```python
from build123d import *

# Parameters (mm, degrees)
SKETCH_1_R          = 25
SKETCH_1_R_2        = 2.55
EXTRUDE_1_DEPTH     = 2
SKETCH_3_R          = 2.05
SKETCH_3_W          = 8.8
SKETCH_3_H          = 2.8
SKETCH_3_W_2        = 2.8
SKETCH_3_H_2        = 8.8
CUT_EXTRUDE_2_DEPTH = 4
SKETCH_7_R          = 3
CUT_EXTRUDE_3_DEPTH = 10
EXTRUDE_3_DEPTH     = 2


with BuildPart() as part:
    # 草图1 → 凸台-拉伸1 (new body)
    with BuildSketch(Plane.XY):
        Polygon((151.457142857, -41.187142857), (151.457142857, 108.812857143), (-148.542857143, 108.812857143), (-148.542857143, -191.187142857), (151.457142857, -191.187142857), align=None)
        with Locations((1.457142857, -41.187142857)):
            Circle(SKETCH_1_R, mode=Mode.SUBTRACT)
        with Locations((25.027142857, -17.617142857)):
            Circle(SKETCH_1_R_2, mode=Mode.SUBTRACT)
        with Locations((25.027142857, -64.757142857)):
            Circle(SKETCH_1_R_2, mode=Mode.SUBTRACT)
        with Locations((-22.112857143, -64.757142857)):
            Circle(SKETCH_1_R_2, mode=Mode.SUBTRACT)
        with Locations((-22.112857143, -17.617142857)):
            Circle(SKETCH_1_R_2, mode=Mode.SUBTRACT)
    extrude(amount=EXTRUDE_1_DEPTH)

    # 草图3 → 切除-拉伸2 (cut)
    with BuildSketch(Plane.XY.offset(2)):
        with Locations((1.457142857, -185.187142857)):
            Circle(SKETCH_3_R)
        with Locations((67.457142857, -185.187142857)):
            Circle(SKETCH_3_R)
        with Locations((-64.542857143, -185.187142857)):
            Circle(SKETCH_3_R)
        with Locations((-142.542857143, 24.812857143)):
            Circle(SKETCH_3_R)
        with Locations((-142.542857143, -41.187142857)):
            Circle(SKETCH_3_R)
        with Locations((-142.542857143, -107.187142857)):
            Circle(SKETCH_3_R)
        with Locations((67.457142857, 102.812857143)):
            Circle(SKETCH_3_R)
        with Locations((1.457142857, 102.812857143)):
            Circle(SKETCH_3_R)
        with Locations((-64.542857143, 102.812857143)):
            Circle(SKETCH_3_R)
        with Locations((145.457142857, -107.187142857)):
            Circle(SKETCH_3_R)
        with Locations((145.457142857, -41.187142857)):
            Circle(SKETCH_3_R)
        with Locations((145.457142857, 24.812857143)):
            Circle(SKETCH_3_R)
        with Locations((50.957142857, -170.187142857)):
            Circle(SKETCH_3_R)
        with Locations((-48.042857143, -170.187142857)):
            Circle(SKETCH_3_R)
        with Locations((1.457142857, -88.187142857)):
            Circle(SKETCH_3_R)
        with Locations((-31.776875859, -74.421161573)):
            Circle(SKETCH_3_R)
        with Locations((-45.542857143, -41.187142857)):
            Circle(SKETCH_3_R)
        with Locations((-31.776875859, -7.953124141)):
            Circle(SKETCH_3_R)
        with Locations((1.457142857, 5.812857143)):
            Circle(SKETCH_3_R)
        with Locations((34.691161573, -7.953124141)):
            Circle(SKETCH_3_R)
        with Locations((48.457142857, -41.187142857)):
            Circle(SKETCH_3_R)
        with Locations((34.691161573, -74.421161573)):
            Circle(SKETCH_3_R)
        with Locations((1.457142857, -125.187142857)):
            Circle(SKETCH_3_R)
        with Locations((100.457142857, -185.187142857)):
            Rectangle(SKETCH_3_W, SKETCH_3_H)
        with Locations((34.457142857, -185.187142857)):
            Rectangle(SKETCH_3_W, SKETCH_3_H)
        with Locations((-31.542857143, -185.187142857)):
            Rectangle(SKETCH_3_W, SKETCH_3_H)
        with Locations((-97.542857143, -185.187142857)):
            Rectangle(SKETCH_3_W, SKETCH_3_H)
        with Locations((-142.542857143, 57.812857143)):
            Rectangle(SKETCH_3_W_2, SKETCH_3_H_2)
        with Locations((-142.542857143, -8.187142857)):
            Rectangle(SKETCH_3_W_2, SKETCH_3_H_2)
        with Locations((-142.542857143, -74.187142857)):
            Rectangle(SKETCH_3_W_2, SKETCH_3_H_2)
        with Locations((-142.542857143, -140.187142857)):
            Rectangle(SKETCH_3_W_2, SKETCH_3_H_2)
        with Locations((100.457142857, 102.812857143)):
            Rectangle(SKETCH_3_W, SKETCH_3_H)
        with Locations((34.457142857, 102.812857143)):
            Rectangle(SKETCH_3_W, SKETCH_3_H)
        with Locations((-31.542857143, 102.812857143)):
            Rectangle(SKETCH_3_W, SKETCH_3_H)
        with Locations((-97.542857143, 102.812857143)):
            Rectangle(SKETCH_3_W, SKETCH_3_H)
        with Locations((145.457142857, -140.187142857)):
            Rectangle(SKETCH_3_W_2, SKETCH_3_H_2)
        with Locations((145.457142857, -74.187142857)):
            Rectangle(SKETCH_3_W_2, SKETCH_3_H_2)
        with Locations((145.457142857, -8.187142857)):
            Rectangle(SKETCH_3_W_2, SKETCH_3_H_2)
        with Locations((145.457142857, 57.812857143)):
            Rectangle(SKETCH_3_W_2, SKETCH_3_H_2)
    extrude(amount=-CUT_EXTRUDE_2_DEPTH, mode=Mode.SUBTRACT)

    # 草图7 → 切除-拉伸3 (cut)
    with BuildSketch(Plane.XY.offset(2)):
        with Locations((-88.542857143, -171.187142857)):
            Circle(SKETCH_7_R)
        with Locations((91.457142857, -171.187142857)):
            Circle(SKETCH_7_R)
        with Locations((-128.542857143, 48.812857143)):
            Circle(SKETCH_7_R)
        with Locations((-128.542857143, -131.187142857)):
            Circle(SKETCH_7_R)
        with Locations((91.457142857, 88.812857143)):
            Circle(SKETCH_7_R)
        with Locations((-88.542857143, 88.812857143)):
            Circle(SKETCH_7_R)
        with Locations((131.457142857, -131.187142857)):
            Circle(SKETCH_7_R)
        with Locations((131.457142857, 48.812857143)):
            Circle(SKETCH_7_R)
    extrude(amount=-CUT_EXTRUDE_3_DEPTH, mode=Mode.SUBTRACT)

    # 草图9 → 凸台-拉伸3 (add)
    with BuildSketch(Plane.XY.offset(2)):
        Polygon((151.457142857, 108.812857143), (251.457142857, 108.812857143), (251.457142857, -191.187142857), (251.457142857, -231.187142857), (-148.542857143, -231.187142857), (-148.542857143, -191.187142857), (151.457142857, -191.187142857), align=None)
    extrude(amount=-EXTRUDE_3_DEPTH)


solid = part.part
```
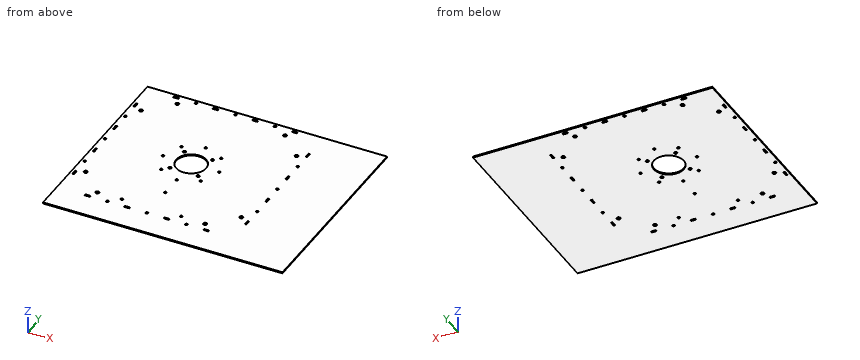
Here's how the part is built. I have some questions about the finished solid (model axes, mm). Coordinates: 2 decimals unless noted, no trailing zeros. Answer as a JSON object with one key per item and string values. Group by question number.
(1) For pin 1 (5.5 mm diameter, centred on x = -142.54, y = -107.19, fed in from -Z); pin 2 (3.5 mm diameter, centred on x = 145.46, y = -107.19, fed in from +Z), each with a flat end and sliding along its axis, tell me the tip position at first contact or that it passes through.
(2) Suppose I cut it at A-A, the plane z = 0.4. State how many separate pieces and enclosed holes the cut face has, then the cut area to 3 significant figures.
(3) I need wall thicknesses on probe 1 along Y at (x, z) = (97, 0.2); probe 2 along X at (y, z) = (58.5, 1.15); probe 3 along X at (y, z) = (6, 0.7). Which ranges of each line are inside material? Lowest first, please.
Values found:
{
 "1": {"pin 1": "stops at z = 0", "pin 2": "passes through"},
 "2": {"separate pieces": "1", "enclosed holes": "52", "area": "133,000 mm^2"},
 "3": {"probe 1": "y = -231.19 to -186.59, -183.79 to 101.41, 104.21 to 108.81", "probe 2": "x = -148.54 to -143.94, -141.14 to 144.06, 146.86 to 251.46", "probe 3": "x = -148.54 to -0.58, 3.5 to 251.46"}
}
